Part model, mm, in its own coordinate system. A direction names the side the tool comes from. Give positions to 0.01 mm unless a question says otherwise; leave off trailing zeros. Order: outer loops, then holes, each group sorted by start corner. A loop starts at its lowest first (then second) coordinate and runs counter-clockwise, first axis right, second up. Notation, with made-up numbers: M 21.25,-7.75 L 73.25,-7.75 A18 cw 73.25,12.25 Z; hole C 70.5,-18.5 d8. An arc over 180 degrees is marked long. Answer as a JSON object with one key per item and string values.
from build123d import *

# Parameters (mm, degrees)
SKETCH4_R           = 24.892
BOSS_EXTRUDE1_DEPTH = 44.45
SKETCH5_R           = 24.892
BOSS_EXTRUDE2_DEPTH = 22.225


with BuildPart() as part:
    # Sketch1 → Revolve1 (revolve)
    with BuildSketch(Plane.XY):
        Polygon((-53.848, -24.892), (-22.225, -24.892), (-22.225, -21.0185), (-53.848, -21.209), align=None)
        Polygon((53.848, -21.209), (22.225, -21.0185), (22.225, -24.892), (53.848, -24.892), align=None)
    revolve(axis=Axis((-53.848, 0, 0), (1, 0, 0)))



with BuildPart() as body_2:
    # Sketch2 → Revolve2 (revolve)
    with BuildSketch(Plane.XY):
        Polygon((21.209, 53.848), (21.0185, 22.225), (24.892, 22.225), (24.892, 53.848), align=None)
    revolve(axis=Axis((0, 0, 0), (0, 1, 0)))


with BuildPart() as part_1:
    add(part.part)

    add(body_2.part)  # Boss-Extrude1 merges body 2
    # Sketch4 → Boss-Extrude1 (add)
    with BuildSketch(Plane(origin=(-22.225, 0, 0), x_dir=(0, 0, -1), z_dir=(1, 0, 0))):
        Circle(SKETCH4_R)
    extrude(amount=BOSS_EXTRUDE1_DEPTH)

    # Sketch5 → Boss-Extrude2 (add)
    with BuildSketch(Plane.XZ.offset(-22.225)):
        Circle(SKETCH5_R)
    extrude(amount=BOSS_EXTRUDE2_DEPTH)

    # Sketch6 → Cut-Revolve1 (revolve, cut)
    with BuildSketch(Plane.XY):
        Polygon((-53.848, -21.209), (-22.225, -21.0185), (-22.225, -17.526), (22.225, -17.526), (22.225, -21.0185), (53.848, -21.209), (53.848, 0), (-53.848, 0), align=None)
    revolve(axis=Axis((53.848, 0, 0), (-1, 0, 0)), mode=Mode.SUBTRACT)

    # Sketch7 → Cut-Revolve2 (revolve, cut)
    with BuildSketch(Plane.XY):
        Polygon((21.209, 53.848), (21.0185, 22.225), (17.526, 22.225), (17.526, 0), (0, 0), (0, 53.848), align=None)
    revolve(axis=Axis((0, 0, 0), (0, 1, 0)), mode=Mode.SUBTRACT)


solid = part_1.part
1. Two-plate mould, pull along Y, no slides. Class faces 3 (the flat face through (18.3, 53.848, -11.2)), 4 (the flat face through (53.848, -18.3, -11.2)), 5 (the cylindrical face through (0.31, -16.19, -6.71)): +Y half, -Y half, draft (parallel to the pull), parting line (faces both ways), or undercut.
Worked answers:
{"face 3": "+Y half", "face 4": "draft", "face 5": "undercut"}
2. Cut at B-B on y = 35. Give the cut face in (x, z).
Worked answers:
{"outline": "C 0,0 d49.78; hole C 0,0 d42.19"}
3. Cut at C-C on x = 38. Give the cut face in (y, z).
Worked answers:
{"outline": "C 0,0 d49.78; hole C 0,0 d42.23"}
4. Probe line 1 along X through (y, z) = (25.5, 0.5); line 2 along Z through (x, y) = (0, 6); line 3 along Y through (x, z) = (10, 0). List the from-to ranges inside material, lowest first.
Worked answers:
{"line 1": "x = -24.89 to -21.03, 21.03 to 24.89", "line 2": "z = -24.89 to -17.53, 17.53 to 24.89", "line 3": "y = -24.89 to -17.53"}
5. Pin check, flat tips, straight feed: P1, Ø5, axis at x = 37, z = 19, coming from the -Y side; P2, Ø1.5, axis at x = 14.5, y = 46, coming from the +Z side; P3, Ø6, axis at x = -17.5, z = -0.5, coming from the +Y side (3 decimals). Stop position of each tip, or through.
Worked answers:
{"P1": "stops at y = -18.64", "P2": "stops at z = 20.75", "P3": "stops at y = 22.225"}
6. Cut at A-A on z = 3.5. State how many separate pieces and enclosed holes the cut face has, plus the area to 3 significant figures.
Worked answers:
{"separate pieces": "3", "enclosed holes": "0", "area": "1,100 mm^2"}
7. Which spindle directions (+Z, -Z, +X, -X, +Y, -Y) get a long thin tool onto all of the face, cutting with end or side? Do faces 1 (the cylindrical face through (-12.92, 15.9, -11.84)), 2 (the flat face through (-53.848, 18.3, -11.2)). Say none if no direction does.
Worked answers:
{"face 1": "+Y", "face 2": "+Z, -Z, -X, +Y, -Y"}
